```python
from build123d import *

# Parameters (mm, degrees)
SKETCH2_W           = 55
SKETCH2_H           = 60
BOSS_EXTRUDE1_DEPTH = 3
SKETCH3_W           = 15
SKETCH3_H           = 25
CUT_EXTRUDE1_DEPTH  = 1
SKETCH4_R           = 1
CUT_EXTRUDE3_DEPTH  = 5
FILLET1_R           = 5
SKETCH5_R           = 1
CUT_EXTRUDE4_DEPTH  = 5
SKETCH6_W           = 15
SKETCH6_H           = 25
CUT_EXTRUDE5_DEPTH  = 1
SKETCH7_R           = 1
CUT_EXTRUDE6_DEPTH  = 2


with BuildPart() as part:
    # Sketch2 → Boss-Extrude1 (new body)
    with BuildSketch(Plane(origin=(0, 0, 0), x_dir=(1, 0, 0), z_dir=(0, 1, 0))):
        with Locations((-50.625, -5.625)):
            Rectangle(SKETCH2_W, SKETCH2_H)
    extrude(amount=BOSS_EXTRUDE1_DEPTH)

    # Sketch3 → Cut-Extrude1 (cut)
    with BuildSketch(Plane(origin=(0, 3, 0), x_dir=(1, 0, 0), z_dir=(0, 1, 0))):
        with Locations((-70.625, -5.625)):
            Rectangle(SKETCH3_W, SKETCH3_H)
    extrude(amount=-CUT_EXTRUDE1_DEPTH, mode=Mode.SUBTRACT)

    # Sketch4 → Cut-Extrude3 (cut)
    with BuildSketch(Plane(origin=(0, 3, 0), x_dir=(1, 0, 0), z_dir=(0, 1, 0))):
        with Locations(Location((-70.625, 2.375, 0), (0, 0, 270))):
            Circle(SKETCH4_R)
        with Locations(Location((-70.625, -13.625, 0), (0, 0, 270))):
            Circle(SKETCH4_R)
    extrude(amount=-CUT_EXTRUDE3_DEPTH, mode=Mode.SUBTRACT)

    # Fillet1
    fillet1_edges = [part.edges().sort_by_distance(p)[0] for p in [
        (-78.125, 1.5, -24.375),
        (-23.125, 1.5, -24.375),
        (-23.125, 1.5, 35.625),
        (-78.125, 1.5, 35.625),
    ]]
    fillet(fillet1_edges, radius=FILLET1_R)

    # Sketch5 → Cut-Extrude4 (cut)
    with BuildSketch(Plane(origin=(0, 3, 0), x_dir=(1, 0, 0), z_dir=(0, 1, 0))):
        with Locations(Location((-50.625, -5.625, 0), (0, 0, 270))):
            Circle(SKETCH5_R)
    extrude(amount=-CUT_EXTRUDE4_DEPTH, mode=Mode.SUBTRACT)

    # Sketch6 → Cut-Extrude5 (cut)
    with BuildSketch(Plane(origin=(0, 3, 0), x_dir=(1, 0, 0), z_dir=(0, 1, 0))):
        with Locations((-30.625, -5.625)):
            Rectangle(SKETCH6_W, SKETCH6_H)
    extrude(amount=-CUT_EXTRUDE5_DEPTH, mode=Mode.SUBTRACT)

    # Sketch7 → Cut-Extrude6 (cut)
    with BuildSketch(Plane(origin=(0, 2, 0), x_dir=(1, 0, 0), z_dir=(0, 1, 0))):
        with Locations(Location((-30.625, 2.375, 0), (0, 0, 270))):
            Circle(SKETCH7_R)
        with Locations(Location((-30.625, -13.625, 0), (0, 0, 270))):
            Circle(SKETCH7_R)
    extrude(amount=-CUT_EXTRUDE6_DEPTH, mode=Mode.SUBTRACT)


solid = part.part
```
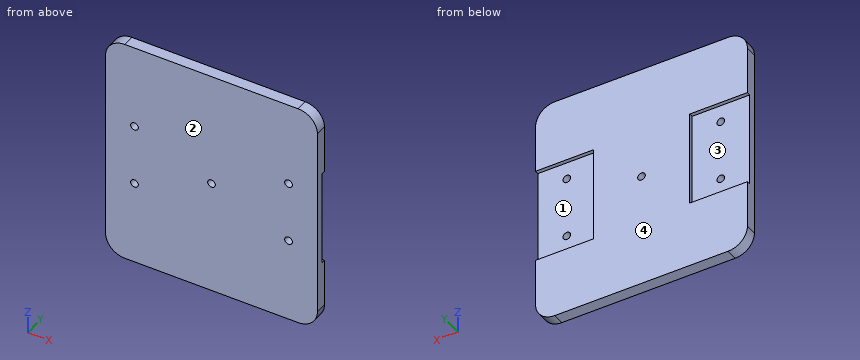
Design review of the part built by this model. Coordinates are the model's own, in mm. Face numbers are marked on the shaded views. A direction names the side the tool comes from. Give positions to 0.01 mm unless a question says otherwise; leave off trailing zeros. Order: outer loops, then holes, each group sorted by start corner. A loop starts at its lowest first (then second) coordinate and runs counter-clockwise, first axis right, second up. Notation, with made-up numbers: M 68,2.5 L 90,2.5 A15 cw 90,25.5 Z; hole C 65.5,66 d5. An arc over 180 degrees is marked long. One line per question, with ' | ' between items. Start each with the question number.
Q1. Machinability: for the marked faces 3 and 4, which of the approach directions +Z, -Z, +X, -X, +Y, -Y give a long, thin tool a straight path to every point of the face, cutting with its end or side? Answer none if there is none.
Q2. We need section A-A (z = 11). Write out the cut boundary in (x, y) (3 decimals).
Q3. The part is to be moulded in two halves that separate along Z. For the marked faces 1 and 2, say which applies: +Z half, -Z half, draft (parallel to the pull), parting line (faces both ways), or undercut.
Q4. For L1, parallel to Z at x = -70, y = 2.4 (3 decimals); L2, parallel to Z at x = -71.5, y = 1.25 (3 decimals); L3, parallel to X at y = 1.9, z = 5.5 (3 decimals), list the stretches that pass through material, from the lowest coordinate up. Write a range as [from, to].
Q5. For pin 1 Ø12 at (x, z) = (-28, 2.5) entering from +Y; pin 2 Ø1.2 at (x, z) = (-30.625, -2.375) entering from -Y, all flat-tipped, find the tip position at first contact; note any pin that passes through.
Q6. We need section B-B (x = -34.5). Write out the cut boundary in (y, z) (3 decimals), plus the area to 3 significant figures.
Returned:
1) face 3: -X, +Y | face 4: +Z, -Z, +X, -X, +Y
2) outline: M -78.125,0 L -23.125,0 L -23.125,2 L -38.125,2 L -38.125,3 L -63.125,3 L -63.125,2 L -78.125,2 Z
3) face 1: undercut | face 2: draft
4) L1: [-24.375, -6.875], [18.125, 35.625] | L2: [-24.375, -2.859], [-1.891, 13.141], [14.109, 35.625] | L3: [-78.125, -51.617], [-49.633, -23.125]
5) pin 1: y = 2 | pin 2: through
6) outline: M 0,-24.375 L 3,-24.375 L 3,-6.875 L 2,-6.875 L 2,18.125 L 3,18.125 L 3,35.625 L 0,35.625 Z | area: 155 mm2
